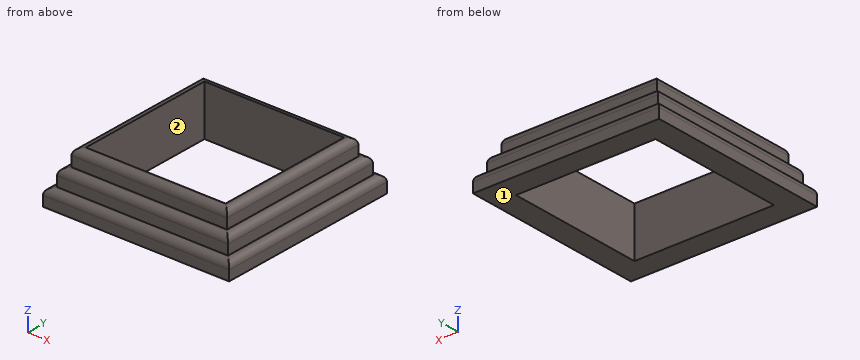
from build123d import *

# Parameters (mm, degrees)
F0_W     = 142.24
F0_H     = 142.24
F1_DEPTH = 12.7
F2_W     = 106.68
F2_H     = 106.68
F3_DEPTH = 12.701
F4_W     = 130.556
F4_H     = 130.556
F4_W_2   = 106.68
F4_H_2   = 106.68
F5_DEPTH = 12.7
F6_W     = 118.872
F6_H     = 118.364
F6_W_2   = 106.68
F6_H_2   = 106.68
F7_DEPTH = 12.7
F8_R     = 5.08


with BuildPart() as f1:
    # F0 (on Top) → F1 (new body)
    with BuildSketch(Plane.XY):
        Rectangle(F0_W, F0_H)
    extrude(amount=F1_DEPTH)

    # F2 (on face) → F3 (cut, through all)
    with BuildSketch(Plane.XY.offset(12.7)):
        Rectangle(F2_W, F2_H)
    extrude(amount=-F3_DEPTH, mode=Mode.SUBTRACT)

    # F4 (on face) → F5 (join)
    with BuildSketch(Plane.XY.offset(12.7)):
        Rectangle(F4_W, F4_H)
        Rectangle(F4_W_2, F4_H_2, mode=Mode.SUBTRACT)
    extrude(amount=F5_DEPTH)

    # F6 (on face) → F7 (join)
    with BuildSketch(Plane.XY.offset(25.4)):
        Rectangle(F6_W, F6_H)
        Rectangle(F6_W_2, F6_H_2, mode=Mode.SUBTRACT)
    extrude(amount=F7_DEPTH)

    # F8
    f8_edges = [f1.edges().sort_by_distance(p)[0] for p in [
        (0, -59.182, 38.1),
        (-59.436, 0, 38.1),
        (0, -65.278, 25.4),
        (0, -71.12, 12.7),
        (-71.12, 0, 12.7),
        (-65.278, 0, 25.4),
        (0, 71.12, 12.7),
        (0, 65.278, 25.4),
        (0, 59.182, 38.1),
        (59.436, 0, 38.1),
        (65.278, 0, 25.4),
        (71.12, 0, 12.7),
    ]]
    fillet(f8_edges, radius=F8_R)


solid = f1.part
Geometry check sheet. Reference: the model listing, model coordinates, mm. Face numbers are marked on the shaded views. Coordinates: 2 decimals unless noted, no trailing zeros. Order: outer loops, then holes, each group sorted by start corner. A loop starts at its lowest first (then second) coordinate and runs counter-clockwise, first axis right, second up. Notation, with made-up numbers: (41.25, 60) - (93.25, 60) arc R23 cw to (93.25, 68) - close; hole circle Ø3 at (25, -14.5). An arc over 180 degrees is marked (long way). Answer in a Markdown table with one row per item. Add a question column.
1) Cross-section at C-C, the plane z = 29.5. Record the cut outline in (x, y), then the cut area to 3 significant figures.
2) Material ranges on line 1 along X through (y, z) = (-10, 18); line 2 along X through (y, z) = (9, 26), recorded low to high. Write a range as [from, to].
3) Cross-section at A-A, the plane x = -17.5. Record the cut outline in (y, z).
4) Cross-section at B-B, the plane y = -28. Record the cut outline in (x, z), then the cut area to 3 significant figures.
5) Gauge pin test, flat ends, axial feed: P1, Ø1, axis at y = 41.5, z = 8.5, coming from the -X side; P2, Ø19, axis at x = -3.5, z = 12, coming from the +Y side; P3, Ø19, axis at x = 18.5, z = 19.5, coming from the -Y side; P4, Ø11.5, axis at y = -20, z = 21.5, coming from the +X side. Record the tip position at first contact, or that the pin passes through.
6) Release check for a two-part mould opening along X. For the marked faces 1 and 2 record: +X half, -X half, draft (parallel to the pull), parting line (faces both ways), or undercut.
Check result:
| question | item | result |
|---|---|---|
| 1 | outline | (-59.44, -59.18) - (59.44, -59.18) - (59.44, 59.18) - (-59.44, 59.18) - close; hole (-53.34, -53.34) - (53.34, -53.34) - (53.34, 53.34) - (-53.34, 53.34) - close |
| 1 | area | 2,690 mm² |
| 2 | line 1 | x = [-65.28, -53.34], [53.34, 65.28] |
| 2 | line 2 | x = [-59.44, -53.34], [53.34, 59.44] |
| 3 | outline | (-71.12, 0) - (-53.34, 0) - (-53.34, 38.1) - (-54.1, 38.1) arc R5.08 ccw to (-59.18, 33.02) - (-59.18, 25.4) - (-60.2, 25.4) arc R5.08 ccw to (-65.28, 20.32) - (-65.28, 12.7) - (-66.04, 12.7) arc R5.08 ccw to (-71.12, 7.62) - close; (53.34, 0) - (71.12, 0) - (71.12, 7.62) arc R5.08 ccw to (66.04, 12.7) - (65.28, 12.7) - (65.28, 20.32) arc R5.08 ccw to (60.2, 25.4) - (59.18, 25.4) - (59.18, 33.02) arc R5.08 ccw to (54.1, 38.1) - (53.34, 38.1) - close |
| 4 | outline | (-71.12, 0) - (-53.34, 0) - (-53.34, 38.1) - (-54.36, 38.1) arc R5.08 ccw to (-59.44, 33.02) - (-59.44, 25.4) - (-60.2, 25.4) arc R5.08 ccw to (-65.28, 20.32) - (-65.28, 12.7) - (-66.04, 12.7) arc R5.08 ccw to (-71.12, 7.62) - close; (53.34, 0) - (71.12, 0) - (71.12, 7.62) arc R5.08 ccw to (66.04, 12.7) - (65.28, 12.7) - (65.28, 20.32) arc R5.08 ccw to (60.2, 25.4) - (59.44, 25.4) - (59.44, 33.02) arc R5.08 ccw to (54.36, 38.1) - (53.34, 38.1) - close |
| 4 | area | 876 mm² |
| 5 | P1 | stops at x = -71.11 |
| 5 | P2 | stops at y = 71.12 |
| 5 | P3 | stops at y = -70.53 |
| 5 | P4 | stops at x = 65.28 |
| 6 | face 1 | draft |
| 6 | face 2 | undercut |
